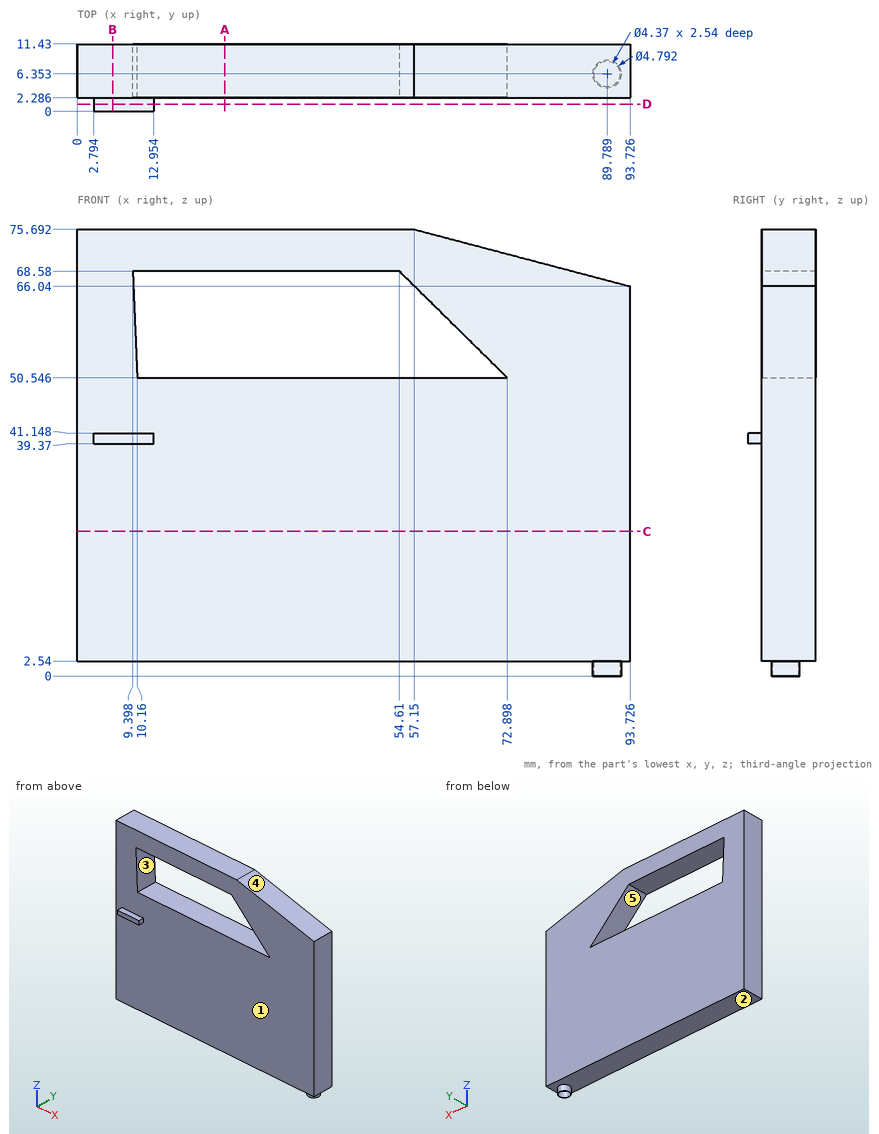
Design review of the part shown in the three views and the two pictorial views. Dimensions are in mm from the part's minimum x, y and z. A direction names the side the tool comes from. Round coordinates to 2 decimals unless told otherwise and drop trailing zeros. Loops run counter-clockwise (first coordinate to the right, second up) from the corner with the lowest first, then second, coordinate; pieces in that order, holes last. Notation, with made-up numbers: M 84,-0.5 L 91,-0.5 A10 ccw 91,6.5 Z; hole C 85,83 d11. An arc over 180 degrees is marked long. Answer as a JSON object with one key per item and string values.
Item 1: We need section A-A on x = 25. Give the boundary of the cut face in (y, z), and give its area (3 significant figures).
Answer sheet:
{"outline": "M 2.29,2.54 L 11.43,2.54 L 11.43,50.55 L 2.29,50.55 Z; M 2.29,68.58 L 11.43,68.58 L 11.43,75.69 L 2.29,75.69 Z", "area": "504 mm^2"}
Item 2: Clearance check with flat-ended pins moving along their axes: P1, Ø2.5, axis at x = 6, y = 1, coming from the -Z side; P2, Ø22, axis at x = 27.5, z = 34.5, coming from the -Y side; P3, Ø4.5, axis at x = 26.5, y = 5.5, coming from the -Z side. State where each tip first meets the part, or that it passes through.
Answer sheet:
{"P1": "stops at z = 39.37", "P2": "stops at y = 2.29", "P3": "stops at z = 2.54"}
Item 3: We need section D-D on y = 1.25. Give the boundary of the cut face in (x, z).
Answer sheet:
{"outline": "M 2.79,39.37 L 12.95,39.37 L 12.95,41.15 L 2.79,41.15 Z"}
Item 4: Machinability: for the marked faces 4 and 5, which of the approach directions +Z, -Z, +X, -X, +Y, -Y give a long, thin tool a straight path to every point of the face, cutting with its end or side? Answer none if there is none.
Answer sheet:
{"face 4": "+Z, +X, +Y, -Y", "face 5": "+Y, -Y"}
Item 5: We need section B-B on x = 6. Give the boundary of the cut face in (y, z).
Answer sheet:
{"outline": "M 0,39.37 L 2.29,39.37 L 2.29,2.54 L 11.43,2.54 L 11.43,75.69 L 2.29,75.69 L 2.29,41.15 L 0,41.15 Z"}
Item 6: We need section C-C on z = 24.5. Give the boundary of the cut face in (x, y), and give its area (3 significant figures).
Answer sheet:
{"outline": "M 0,2.29 L 93.73,2.29 L 93.73,11.43 L 0,11.43 Z", "area": "857 mm^2"}
Item 7: Wall thickness on L1, parallel to Z at x = 39, y = 7; L2, parallel to Y at x = 34, z = 7; L3, parallel to X at y = 10.25, z = 58.5 (1 decimal): over which ranges is each line inside the solid? List them lowest first. Write a range as from..to.
Answer sheet:
{"L1": "z = 2.54..50.55, 68.58..75.69", "L2": "y = 2.29..11.43", "L3": "x = 0..9.8, 64.8..93.7"}
Item 8: The part is to be moulded in two halves that separate along Z. For the marked faces 1, 2 and 3, say which applies: pulls with the +Z half, pulls with the -Z half, needs draft (parallel to the pull), parting line crosses it, or undercut.
Answer sheet:
{"face 1": "needs draft", "face 2": "pulls with the -Z half", "face 3": "undercut"}
